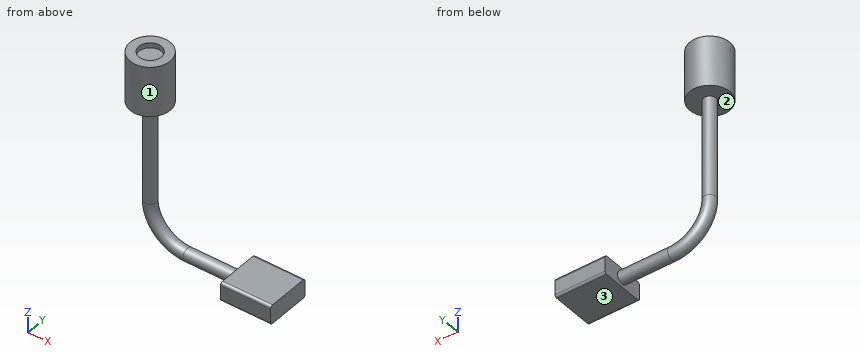
```python
from build123d import *

# Parameters (mm, degrees)
SKETCH_R     = 8
PAD_DEPTH    = 20
SKETCH002_R  = 2.5
SKETCH003_R  = 4.5
POCKET_DEPTH = 2
PAD001_DEPTH = 20


with BuildPart() as part:
    # Sketch → Pad (new body)
    with BuildSketch(Plane.XY):
        Circle(SKETCH_R)
    extrude(amount=PAD_DEPTH)

    # AdditivePipe: sweep along a path in Sketch001
    with BuildLine(Plane.XZ) as additivepipe_path:
        Line((0, 0), (0, -40))
        ThreePointArc((0, -40), (4.393398, -50.606602), (15, -55))
        Line((15, -55), (35, -55))
    # Sketch002 (on Face2 of Pad) → AdditivePipe (sweep)
    with BuildSketch(Plane(origin=(0, 0, 0), x_dir=(1, 0, 0), z_dir=(0, 0, -1))):
        Circle(SKETCH002_R)
    sweep(path=additivepipe_path.line)

    # Sketch003 (on Face3 of AdditivePipe) → Pocket (cut)
    with BuildSketch(Plane.XY.offset(20)):
        Circle(SKETCH003_R)
    extrude(amount=-POCKET_DEPTH, mode=Mode.SUBTRACT)

    # Sketch004 (on Face9 of Pocket) → Pad001 (join)
    with BuildSketch(Plane.YZ.offset(35)):
        with BuildLine():
            Line((-9, -52.301853), (-9, -57.925102))
            ThreePointArc((-9, -57.925102), (-8.758393, -58.508393), (-8.175102, -58.75))
            Line((-8.175102, -58.75), (8.209949, -58.75))
            ThreePointArc((8.209949, -58.75), (8.7686, -58.5186), (9, -57.959949))
            Line((9, -57.959949), (9, -52.278293))
            ThreePointArc((9, -52.278293), (8.69882, -51.55118), (7.971707, -51.25))
            Line((7.971707, -51.25), (-7.948147, -51.25))
            ThreePointArc((-7.948147, -51.25), (-8.691919, -51.558081), (-9, -52.301853))
        make_face()
    extrude(amount=PAD001_DEPTH)


solid = part.part
```
For this review, take the finished solid that the model builds, in its own axes (mm). Face numbers are marked on the shaded views. Round coordinates to 2 decimals unless told otherwise and drop trailing zeros. Write each loop counter-clockwise with the first axis right and the second up, starting at its lowest first coordinate (ties: lowest second). Pieces come first, ordered by that corner, then holes. Notation, with made-up numbers: M 49.5,21.25 L 94.5,21.25 A15 cw 94.5,44.25 Z; hole C 11.25,-12 d5. An arc over 180 degrees is marked long. One line per item, written item: value. Start each with the question number.
(1) The part is to be moulded in two halves that separate along Z. For the marked faces 1, 2 and 3, say which applies: released by +Z, released by -Z, zero draft, split by the parting line, or undercut.
(2) We need section B-B (z = 15.5). Give the boundary of the cut face in (x, y), and give its area (3 significant figures).
(3) We need section C-C (z = -13.5). Give the boundary of the cut face in (x, y), and give its area (3 significant figures).
(4) Insertion check: pin 1 (3 mm diameter, centred on y = 0.5, z = 11.5, fed in from +X); pin 2 (6 mm diameter, centred on y = -2.5, z = -55, fed in from -X); pin 3 (8 mm diameter, centred on x = -2, y = 0.5, fed in from -Z). Each pin has a flat end and moves straight along its axis. Give the tip position at first contact, or say it passes through.
(5) We need section A-A (x = 47.5). Give the boundary of the cut face in (y, z), and give its area (3 significant figures).
(6) Wall thickness on line 1 (Y direction, x = 0, z = 19.4); line 2 (Z direction, x = 46, y = -3.75); line 3 (Z direction, x = 0, y = 4.25): over which ranges is each line inside the solid? List them lowest first.
Result:
1. face 1: zero draft
1. face 2: undercut
1. face 3: released by -Z
2. outline: C 0,0 d16
2. area: 201 mm²
3. outline: C 0,0 d5
3. area: 19.6 mm²
4. pin 1: x = 8
4. pin 2: x = 2.95
4. pin 3: z = -51.69
5. outline: M -9,-57.93 A0.82 ccw -8.18,-58.75 L 8.21,-58.75 A0.79 ccw 9,-57.96 L 9,-52.28 A1.03 ccw 7.97,-51.25 L -7.95,-51.25 A1.05 ccw -9,-52.3 Z
5. area: 134 mm²
6. line 1: -8 to -4.5, 4.5 to 8
6. line 2: -58.75 to -51.25
6. line 3: 0 to 18
